Source: CAD feature listing. Evaluate the final solid. Frame: model axes, mm. Face numbers are marked on the shaded views. A direction names the side the tool comes from. Round coordinates to 2 decimals unless told otherwise and drop trailing zeros. Write each loop counter-clockwise with the first axis right and the second up, starting at its lowest first coordinate (ties: lowest second). Pieces come first, ordered by that corner, then holes.
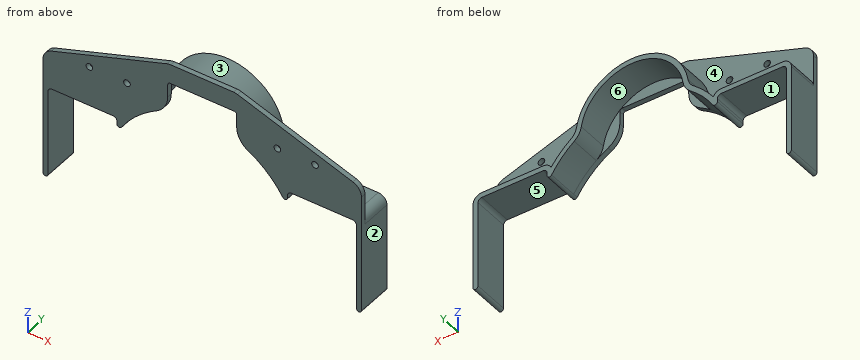
```python
from build123d import *

# Parameters (mm, degrees)
SKETCH_2_R      = 2.65
EXTRUDE_1_DEPTH = 4
EXTRUDE_2_DEPTH = 25


with BuildPart() as part:
    # 草图2 → 凸台-拉伸1 (new body)
    # profile 1 of 5: a face of its own
    with BuildSketch(Plane(origin=(0, 0, 0), x_dir=(1, 0, 0), z_dir=(0, 1, 0))):
        with BuildLine():
            Line((-27.5, 2), (-27.5, 12.147710197))
            ThreePointArc((-27.5, 12.147710197), (-29.994681763, 21.290199266), (-36.787234043, 27.898510474))
            ThreePointArc((-36.787234043, 27.898510474), (-38.913878838, 29.12011529), (-41, 30.409702399))
            ThreePointArc((-41, 30.409702399), (-53.947743005, 40.870206984), (-64.307692308, 53.898547461))
            ThreePointArc((-64.307692308, 53.898547461), (-66.554700196, 54.754207886), (-68, 52.832670041))
            Line((-68, 52.832670041), (-68, 50.409702399))
            ThreePointArc((-68, 50.409702399), (-68.878679656, 48.288382056), (-71, 47.409702399))
            Line((-71, 47.409702399), (-120, 47.409702399))
            ThreePointArc((-120, 47.409702399), (-122.121320344, 48.288382056), (-123, 50.409702399))
            Line((-123, 50.409702399), (-123, 119.409702399))
            ThreePointArc((-123, 119.409702399), (-125, 121.409702399), (-127, 119.409702399))
            Line((-127, 119.409702399), (-127, 25.409702399))
            ThreePointArc((-127, 25.409702399), (-125.121934023, 19.575819668), (-120.193162456, 15.933220271))
            Line((-120.193162456, 15.933220271), (-90, 5.759437269))
            Line((-90, 5.759437269), (-90, 12.759702399))
            ThreePointArc((-90, 12.759702399), (-91.87383297, 17.283535369), (-87.35, 15.409702399))
            Line((-87.35, 15.409702399), (-62.65, 15.409702399))
            ThreePointArc((-62.65, 15.409702399), (-60, 18.059702399), (-57.35, 15.409702399))
            ThreePointArc((-57.35, 15.409702399), (-58.12616703, 13.535869429), (-60, 12.759702399))
            Line((-60, 12.759702399), (-60, -4.349258383))
            Line((-60, -4.349258383), (-28.193162456, -15.066779729))
            ThreePointArc((-28.193162456, -15.066779729), (-26.617896585, -15.458550265), (-25, -15.590297601))
            Line((-25, -15.590297601), (25, -15.590297601))
            ThreePointArc((25, -15.590297601), (26.617896585, -15.458550265), (28.193162456, -15.066779729))
            Line((28.193162456, -15.066779729), (120.193162456, 15.933220271))
            ThreePointArc((120.193162456, 15.933220271), (125.121934023, 19.575819668), (127, 25.409702399))
            Line((127, 25.409702399), (127, 119.409702399))
            ThreePointArc((127, 119.409702399), (125, 121.409702399), (123, 119.409702399))
            Line((123, 119.409702399), (123, 50.409702399))
            ThreePointArc((123, 50.409702399), (122.121320344, 48.288382056), (120, 47.409702399))
            Line((120, 47.409702399), (71, 47.409702399))
            ThreePointArc((71, 47.409702399), (68.878679656, 48.288382056), (68, 50.409702399))
            Line((68, 50.409702399), (68, 52.832670041))
            ThreePointArc((68, 52.832670041), (66.554700196, 54.754207886), (64.307692308, 53.898547461))
            ThreePointArc((64.307692308, 53.898547461), (52.192399009, 39.157401138), (36.787234043, 27.898510474))
            ThreePointArc((36.787234043, 27.898510474), (29.994681763, 21.290199266), (27.5, 12.147710197))
            Line((27.5, 12.147710197), (27.5, 2))
            ThreePointArc((27.5, 2), (26.914213562, 0.585786438), (25.5, 0))
            Line((25.5, 0), (-25.5, 0))
            ThreePointArc((-25.5, 0), (-26.914213562, 0.585786438), (-27.5, 2))
        make_face()
        with Locations(Location((60, 15.409702399, 0), (0, 0, 270))):
            Circle(SKETCH_2_R, mode=Mode.SUBTRACT)
        with Locations(Location((90, 15.409702399, 0), (0, 0, 270))):
            Circle(SKETCH_2_R, mode=Mode.SUBTRACT)
    # profile 2 of 5: a face of its own
    with BuildSketch(Plane(origin=(0, 0, 0), x_dir=(1, 0, 0), z_dir=(0, 1, 0))):
        with BuildLine():
            Line((-90, 12.759702399), (-90, 5.759437269))
            Line((-90, 5.759437269), (-77.378818279, 1.506647776))
            Line((-77.378818279, 1.506647776), (-75, 3.409702399))
            Line((-75, 3.409702399), (-87.930697655, 13.754260523))
            ThreePointArc((-87.930697655, 13.754260523), (-88.852049864, 13.021248823), (-90, 12.759702399))
        make_face()
    # profile 3 of 5: a face of its own
    with BuildSketch(Plane(origin=(0, 0, 0), x_dir=(1, 0, 0), z_dir=(0, 1, 0))):
        with BuildLine():
            Line((-87.930697655, 13.754260523), (-75, 3.409702399))
            Line((-75, 3.409702399), (-62.069302345, 13.754260523))
            ThreePointArc((-62.069302345, 13.754260523), (-62.500615046, 14.532534004), (-62.65, 15.409702399))
            Line((-62.65, 15.409702399), (-87.35, 15.409702399))
            ThreePointArc((-87.35, 15.409702399), (-87.499384954, 14.532534004), (-87.930697655, 13.754260523))
        make_face()
    # profile 4 of 5: a face of its own
    with BuildSketch(Plane(origin=(0, 0, 0), x_dir=(1, 0, 0), z_dir=(0, 1, 0))):
        with BuildLine():
            Line((-75, 3.409702399), (-69.159051832, -1.263056135))
            Line((-69.159051832, -1.263056135), (-60, -4.349258383))
            Line((-60, -4.349258383), (-60, 12.759702399))
            ThreePointArc((-60, 12.759702399), (-61.147950136, 13.021248823), (-62.069302345, 13.754260523))
            Line((-62.069302345, 13.754260523), (-75, 3.409702399))
        make_face()
    # profile 5 of 5: a face of its own
    with BuildSketch(Plane(origin=(0, 0, 0), x_dir=(1, 0, 0), z_dir=(0, 1, 0))):
        Polygon((-75, 3.409702399), (-77.378818279, 1.506647776), (-69.159051832, -1.263056135), align=None)
    extrude(amount=EXTRUDE_1_DEPTH)

    # 草图3 → 凸台-拉伸2 (add)
    with BuildSketch(Plane(origin=(0, 4, 0), x_dir=(1, 0, 0), z_dir=(0, 1, 0))):
        with BuildLine():
            Line((127, 50.409702399), (127, 115.409702399))
            Line((127, 115.409702399), (127, 119.409702399))
            ThreePointArc((127, 119.409702399), (125, 121.409702399), (123, 119.409702399))
            Line((123, 119.409702399), (123, 50.409702399))
            ThreePointArc((123, 50.409702399), (122.121320344, 48.288382056), (120, 47.409702399))
            Line((120, 47.409702399), (71, 47.409702399))
            ThreePointArc((71, 47.409702399), (68.878679656, 48.288382056), (68, 50.409702399))
            Line((68, 50.409702399), (68, 52.832670041))
            ThreePointArc((68, 52.832670041), (66.554700196, 54.754207886), (64.307692308, 53.898547461))
            ThreePointArc((64.307692308, 53.898547461), (56.167018952, 43.203588844), (46.269641343, 34.109930672))
            ThreePointArc((46.269641343, 34.109930672), (42.548019366, 29.9419633), (40.610070261, 24.701087856))
            ThreePointArc((40.610070261, 24.701087856), (0, -9.642140289), (-40.610070261, 24.701087856))
            ThreePointArc((-40.610070261, 24.701087856), (-42.548019366, 29.9419633), (-46.269641343, 34.109930672))
            ThreePointArc((-46.269641343, 34.109930672), (-56.167018952, 43.203588844), (-64.307692308, 53.898547461))
            ThreePointArc((-64.307692308, 53.898547461), (-66.554700196, 54.754207886), (-68, 52.832670041))
            Line((-68, 52.832670041), (-68, 50.409702399))
            ThreePointArc((-68, 50.409702399), (-68.878679656, 48.288382056), (-71, 47.409702399))
            Line((-71, 47.409702399), (-120, 47.409702399))
            ThreePointArc((-120, 47.409702399), (-122.121320344, 48.288382056), (-123, 50.409702399))
            Line((-123, 50.409702399), (-123, 119.409702399))
            ThreePointArc((-123, 119.409702399), (-125, 121.409702399), (-127, 119.409702399))
            Line((-127, 119.409702399), (-127, 115.409702399))
            Line((-127, 115.409702399), (-127, 50.409702399))
            ThreePointArc((-127, 50.409702399), (-124.949747468, 45.459954931), (-120, 43.409702399))
            Line((-120, 43.409702399), (-71, 43.409702399))
            ThreePointArc((-71, 43.409702399), (-67.284863149, 44.476932542), (-64.702556592, 47.353200063))
            ThreePointArc((-64.702556592, 47.353200063), (-57.294743258, 38.568992354), (-48.704885624, 30.936669685))
            ThreePointArc((-48.704885624, 30.936669685), (-45.975696175, 27.880160279), (-44.554533498, 24.03685162))
            ThreePointArc((-44.554533498, 24.03685162), (0, -13.642140289), (44.554533498, 24.03685162))
            ThreePointArc((44.554533498, 24.03685162), (45.975696175, 27.880160279), (48.704885624, 30.936669685))
            ThreePointArc((48.704885624, 30.936669685), (57.294743258, 38.568992354), (64.702556592, 47.353200063))
            ThreePointArc((64.702556592, 47.353200063), (67.284863149, 44.476932542), (71, 43.409702399))
            Line((71, 43.409702399), (120, 43.409702399))
            ThreePointArc((120, 43.409702399), (124.949747468, 45.459954931), (127, 50.409702399))
        make_face()
    extrude(amount=EXTRUDE_2_DEPTH)


solid = part.part
```
Q1. Set-up query: the marked faces 4, 5 and 6. Return all of +Z, -Z, +X, -X, +Y, -Y with unobstructed straight access to the full face (end or side cutting, diameter ignored); none if empty.
Q2. Mould query, pull axis X, two halves, no side actions, for the marked faces 1, 2 and 3. Classes: pulls with the +X half, pulls with the -X half, needs draft (parallel to the pull), parting line crosses it, or undercut.
Q3. Line query: line 1 (X direction, y = 22.5, z = -67); line 2 (Z direction, x = -111, y = 17.5); line 3 (Y direction, x = -51.5, z = -20). Output: solid intervals per line, ascending.
Q4. Pin query (flat end, axial travel): P1, Ø1, axis at x = 53, y = 15, coming from the -Z side; P2, Ø7, axis at x = 60, z = -15.41, coming from the +Y side; P3, Ø8, axis at x = 64, y = 15.5, coming from the +Z side. Return the tip coordinate at first contact, or that it passes through.
Q5. Section query D-D, the plane x = 16. Output: boundary loops of the cut face in (y, z), and give its area (3 significant figures).
Q6. Section query A-A, the plane x = 90. Output: boundary loops of the cut face in (y, z).
Q7. Section query C-C, the plane z = -21. Output: boundary loops of the cut face in (x, y), and give its area (3 significant figures).
Filled in:
1. face 4: +Z, +Y
1. face 5: -Z, +Y, -Y
1. face 6: -Z, +Y
2. face 1: undercut
2. face 2: pulls with the +X half
2. face 3: parting line crosses it
3. line 1: x = -127 to -123, 123 to 127
3. line 2: z = -47.41 to -43.41
3. line 3: y = 0 to 4
4. P1: stops at z = -40.42
4. P2: stops at y = 4
4. P3: stops at z = -41.49
5. outline: (0, 0) - (4, 0) - (4, 6.41) - (29, 6.41) - (29, 10.71) - (4, 10.71) - (4, 15.59) - (0, 15.59) - close
5. area: 170 mm2
6. outline: (0, -47.41) - (29, -47.41) - (29, -43.41) - (4, -43.41) - (4, -18.06) - (0, -18.06) - close; (0, -12.76) - (4, -12.76) - (4, -5.76) - (0, -5.76) - close
7. outline: (-125.98, 0) - (-29.83, 0) - (-29.83, 4) - (-39.81, 4) - (-39.81, 29) - (-43.94, 29) - (-43.94, 4) - (-125.98, 4) - close; (29.83, 0) - (125.98, 0) - (125.98, 4) - (43.94, 4) - (43.94, 29) - (39.81, 29) - (39.81, 4) - (29.83, 4) - close
7. area: 975 mm2
